Verification items for this drawing (mm, ordinates from the low corner). Coordinates: 2 decimals unless noted, no trailing zeros. Write each loop counter-clockwise with the first axis right and the second up, starting at its lowest first coordinate (ties: lowest second). Pieces come first, ordered by that corner, then holes.
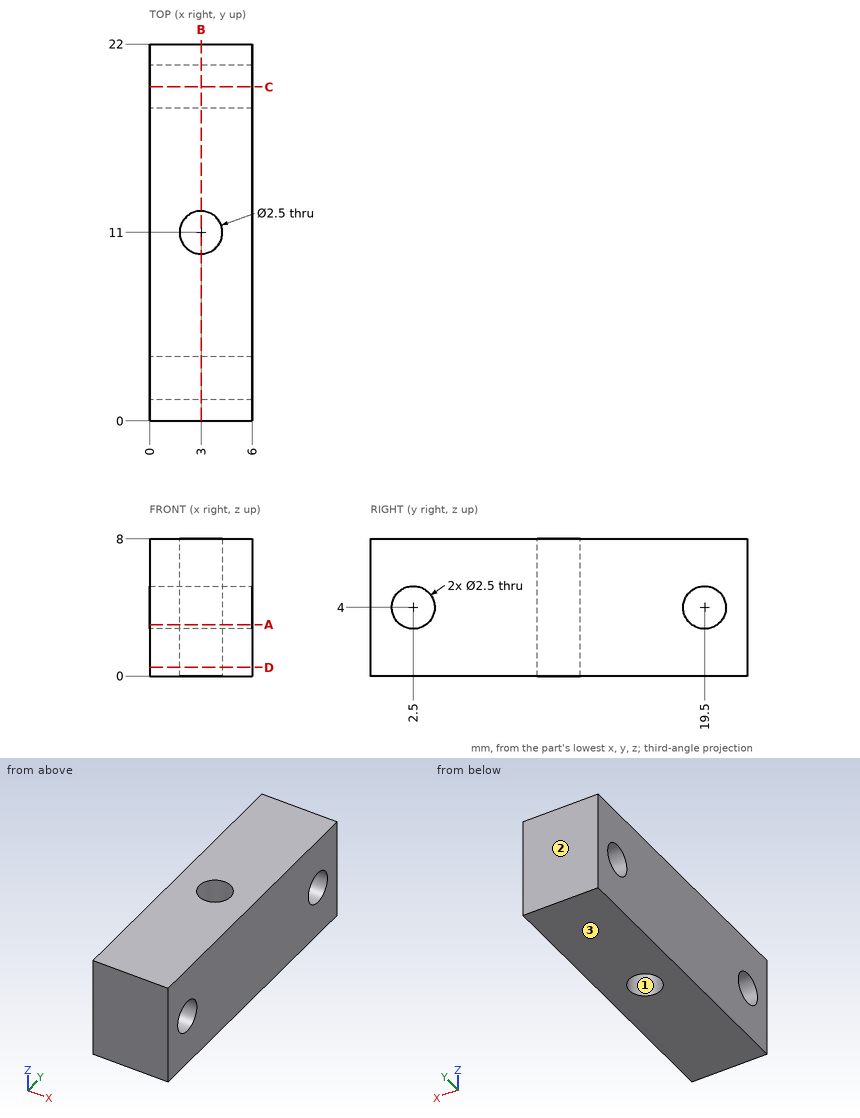
1. Thickness scan on line 1 along Y through (x, z) = (3, 4); line 2 along Y through (x, z) = (4.6, 4); line 3 along Y through (x, z) = (4.3, 5). Record the ranges inside material, lowest first.
Computed values:
line 1: y = 0 to 1.25, 3.75 to 9.75, 12.25 to 18.25, 20.75 to 22
line 2: y = 0 to 1.25, 3.75 to 18.25, 20.75 to 22
line 3: y = 0 to 1.75, 3.25 to 18.75, 20.25 to 22
2. Sectioned sample at B-B, the plane x = 3. Record the boundary of the cut face in (y, z), and give its area (3 significant figures).
Computed values:
outline: (0, 0) - (9.75, 0) - (9.75, 8) - (0, 8) - close; (12.25, 0) - (22, 0) - (22, 8) - (12.25, 8) - close; hole circle Ø2.5 at (2.5, 4); hole circle Ø2.5 at (19.5, 4)
area: 146 mm2
3. Sectioned sample at A-A, the plane z = 3. Record the boundary of the cut face in (x, y), and give its area (3 significant figures).
Computed values:
outline: (0, 0) - (6, 0) - (6, 1.75) - (0, 1.75) - close; (0, 3.25) - (6, 3.25) - (6, 18.75) - (0, 18.75) - close; (0, 20.25) - (6, 20.25) - (6, 22) - (0, 22) - close; hole circle Ø2.5 at (3, 11)
area: 109 mm2
4. Sectioned sample at C-C, the plane y = 19.5. Record the boundary of the cut face in (x, z).
Computed values:
outline: (0, 0) - (6, 0) - (6, 2.75) - (0, 2.75) - close; (0, 5.25) - (6, 5.25) - (6, 8) - (0, 8) - close
5. Draft check along Y on the marked faces 1, 2 and 3. Enter one of: released by +Y, released by -Y, zero draft, split by the parting line, or undercut.
Computed values:
face 1: undercut
face 2: released by +Y
face 3: zero draft
6. Gauge pin test, flat end, axial feed: pin 1 Ø2 at (x, y) = (3, 11) entering from -Z. Record the tip position at first contact, or that the pin passes through.
Computed values:
pin 1: passes through
7. Sectioned sample at D-D, the plane z = 0.5. Record the boundary of the cut face in (x, y).
Computed values:
outline: (0, 0) - (6, 0) - (6, 22) - (0, 22) - close; hole circle Ø2.5 at (3, 11)
